```python
from build123d import *

# Parameters (mm, degrees)
SKETCH_282_W          = 10
SKETCH_282_H          = 10
SKETCH_282_W_2        = 8
SKETCH_282_H_2        = 8
EXTRUDE_339_DEPTH     = 90
SKETCH_411_R          = 1.6
CUT_EXTRUDE_834_DEPTH = 91.691785736
SKETCH_636_R          = 1.6
CUT_EXTRUDE_878_DEPTH = 91.691785736


with BuildPart() as part:
    # Sketch 282 → Extrude 339 (new body)
    with BuildSketch(Plane.XY):
        Rectangle(SKETCH_282_W, SKETCH_282_H)
        Rectangle(SKETCH_282_W_2, SKETCH_282_H_2, mode=Mode.SUBTRACT)
    extrude(amount=EXTRUDE_339_DEPTH)

    # Sketch 411 → Cut-Extrude 834 (cut, through all)
    with BuildSketch(Plane(origin=(0, 5, 0), x_dir=(1, 0, 0), z_dir=(0, 1, 0))):
        with Locations(Location((0, -5, 0), (0, 0, 270))):
            Circle(SKETCH_411_R)
        with Locations(Location((0, -85, 0), (0, 0, 270))):
            Circle(SKETCH_411_R)
        with Locations(Location((0, -13, 0), (0, 0, 270))):
            Circle(SKETCH_411_R)
        with Locations(Location((0, -77, 0), (0, 0, 270))):
            Circle(SKETCH_411_R)
    extrude(amount=-CUT_EXTRUDE_834_DEPTH, mode=Mode.SUBTRACT)

    # Sketch 636 → Cut-Extrude 878 (cut, through all)
    with BuildSketch(Plane(origin=(5, 0, 0), x_dir=(0, 0, -1), z_dir=(1, 0, 0))):
        with Locations((-27.5, 0)):
            Circle(SKETCH_636_R)
        with Locations((-62.5, 0)):
            Circle(SKETCH_636_R)
    extrude(amount=-CUT_EXTRUDE_878_DEPTH, mode=Mode.SUBTRACT)


solid = part.part
```
Verification items for the finished model (mm, model axes). A direction names the side the tool comes from. Give positions to 0.01 mm unless a question says otherwise; leave off trailing zeros. Order: outer loops, then holes, each group sorted by start corner. A loop starts at its lowest first (then second) coordinate and runs counter-clockwise, first axis right, second up. Notation, with made-up numbers: M 23.5,62.5 L 41.5,62.5 A14 ccw 41.5,85.5 Z; hole C 63.5,13.25 d1. An arc over 180 degrees is marked long. Return JSON: item names as keys, results as strings. Group by question number.
1) Go/stop test with flat-tipped pins: pin 1 Ø4 at (x, y) = (0.5, -0.5) entering from +Z; pin 2 Ø5 at (y, z) = (0, 27.5) entering from +X. Record where each tip stops, or that it passes through.
2) Section check B-B on x = 2.5. Record the cut outline in (y, z).
3) Access from +Z, -Z, +X, -X, +Y, -Y to the whole of each face (thin tool, end or side, straight path). Record for faces 1 (the face through (-4.49, 1.08, 28.68)), 2 (the face through (0, 4, 44)).
4) Mould release check, pull along X, two halves, no side actions. Record for faces 3 (the face through (-5, 0, 44)), 4 (the face through (-0.61, 4.51, 6.48)), 5 (the face through (-4.5, 0.1, 0)): pulls with the +X half, pulls with the -X half, needs draft (parallel to the pull), parting line crosses it, or undercut.
5) Section check A-A on z = 77. Record the cut outline in (x, y), and give its area (3 significant figures).
6) Section check C-C on y = 0. Record the cut outline in (x, z).
7) Scan lines: line 1 (X direction, y = -4.8, z = 77); line 2 (X direction, y = -1.5, z = 57.5). Record each from-to range of solid material in increasing order.
Answer block:
{
 "1": {"pin 1": "passes through", "pin 2": "stops at x = 5"},
 "2": {"outline": "M -5,0 L -4,0 L -4,90 L -5,90 Z; M 4,0 L 5,0 L 5,90 L 4,90 Z"},
 "3": {"face 1": "+X, -X", "face 2": "+Z, -Z"},
 "4": {"face 3": "pulls with the -X half", "face 4": "undercut", "face 5": "needs draft"},
 "5": {"outline": "M -5,-5 L -1.6,-5 L -1.6,-4 L -4,-4 L -4,4 L -1.6,4 L -1.6,5 L -5,5 Z; M 1.6,-5 L 5,-5 L 5,5 L 1.6,5 L 1.6,4 L 4,4 L 4,-4 L 1.6,-4 Z", "area": "29.6 mm^2"},
 "6": {"outline": "M -5,0 L -4,0 L -4,25.9 L -5,25.9 Z; M -5,29.1 L -4,29.1 L -4,60.9 L -5,60.9 Z; M -5,64.1 L -4,64.1 L -4,90 L -5,90 Z; M 4,0 L 5,0 L 5,25.9 L 4,25.9 Z; M 4,29.1 L 5,29.1 L 5,60.9 L 4,60.9 Z; M 4,64.1 L 5,64.1 L 5,90 L 4,90 Z"},
 "7": {"line 1": "x = -5 to -1.6, 1.6 to 5", "line 2": "x = -5 to -4, 4 to 5"}
}
